Here's the drawing with two shaded views (mm, measured from the low corner). I have some questions. A direction names the side the tool comes from. Round coordinates to 2 decimals unless told otherwise and drop trailing zeros. Loops run counter-clockwise (first coordinate to the right, second up) from the corner with the lowest first, then second, coordinate; pieces in that order, holes last. Notation, with made-up numbers: (68, 36.25) -> (102, 36.25) arc R21 cw to (102, 41.25) -> close; hole circle Ø11 at (-17, 68.5). An arc over 180 degrees is marked (long way). Use a Markdown table: item, result.
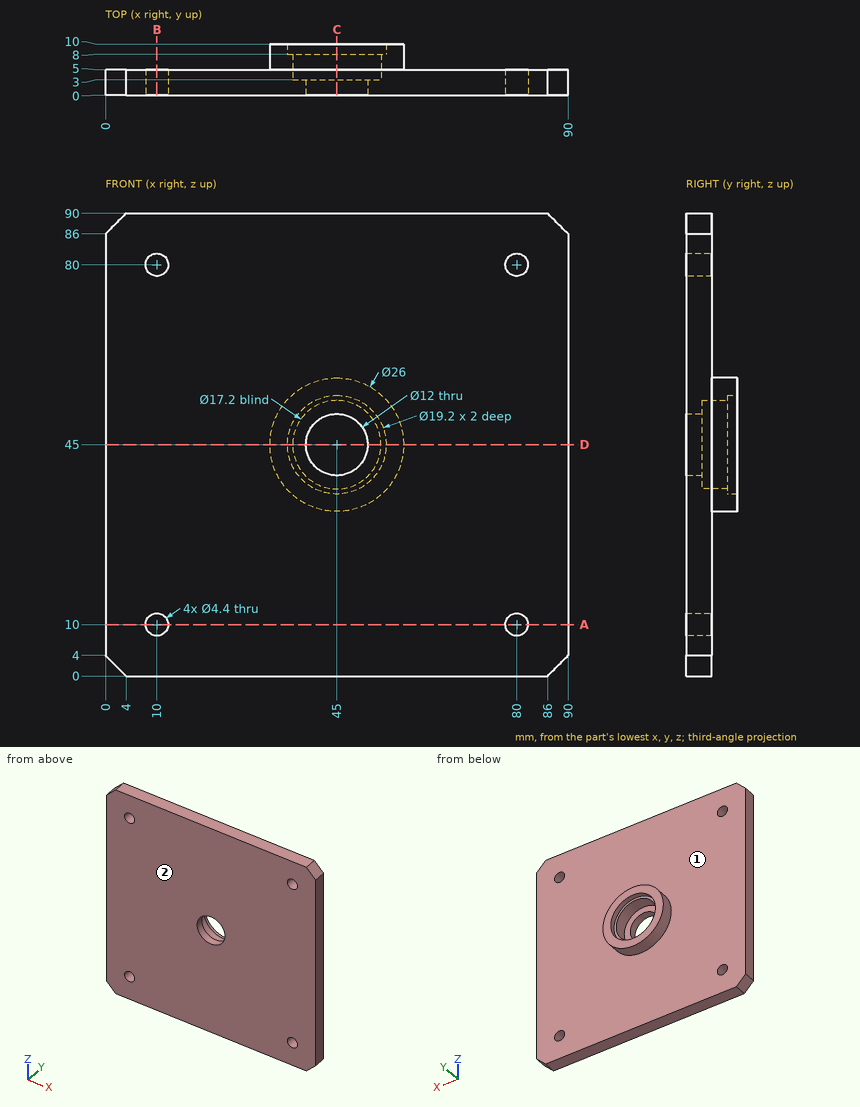
1. I want a section at A-A (z = 10). Please give me the cut outline in (x, y).
Answer sheet:
| item | result |
|---|---|
| outline | (0, 0) -> (7.8, 0) -> (7.8, 5) -> (0, 5) -> close; (12.2, 0) -> (77.8, 0) -> (77.8, 5) -> (12.2, 5) -> close; (82.2, 0) -> (90, 0) -> (90, 5) -> (82.2, 5) -> close |
2. I want a section at C-C (x = 45). Please give me the cut outline in (y, z), plus the area to 3 significant figures.
Answer sheet:
| item | result |
|---|---|
| outline | (0, 0) -> (5, 0) -> (5, 32) -> (10, 32) -> (10, 35.4) -> (8, 35.4) -> (8, 36.4) -> (3, 36.4) -> (3, 39) -> (0, 39) -> close; (0, 51) -> (3, 51) -> (3, 53.6) -> (8, 53.6) -> (8, 54.6) -> (10, 54.6) -> (10, 58) -> (5, 58) -> (5, 90) -> (0, 90) -> close |
| area | 420 mm² |
3. Which directions (+Z, -Z, +X, -X, +Y, -Y) give clear straight access to the entire face, cutting with the end or side of a thin tool? Please do the marked faces 1 and 2.
Answer sheet:
| item | result |
|---|---|
| face 1 | +Y |
| face 2 | +Z, -Z, +X, -X, -Y |
4. I want a section at D-D (z = 45). Please give me the cut outline in (x, y), plus the area to 3 significant figures.
Answer sheet:
| item | result |
|---|---|
| outline | (0, 0) -> (39, 0) -> (39, 3) -> (36.4, 3) -> (36.4, 8) -> (35.4, 8) -> (35.4, 10) -> (32, 10) -> (32, 5) -> (0, 5) -> close; (51, 0) -> (90, 0) -> (90, 5) -> (58, 5) -> (58, 10) -> (54.6, 10) -> (54.6, 8) -> (53.6, 8) -> (53.6, 3) -> (51, 3) -> close |
| area | 420 mm² |
5. Will these pins go through, and if not, where does the flat tip stop? pin 1 Ø9.5 at (x, z) = (41, 46.5) entering from +Y; pin 2 Ø2 at (y, z) = (7.5, 69.5) entering from +X.
Answer sheet:
| item | result |
|---|---|
| pin 1 | stops at y = 8 |
| pin 2 | passes through |
6. I need wall thicknesses on line 1 (X direction, y = 2.7, z = 10); line 2 (X direction, y = 9.1, z = 45); line 3 (X direction, y = 2.2, z = 45). Which ranges of each line are inside material? Lowest first, please.
Answer sheet:
| item | result |
|---|---|
| line 1 | x = 0 to 7.8, 12.2 to 77.8, 82.2 to 90 |
| line 2 | x = 32 to 35.4, 54.6 to 58 |
| line 3 | x = 0 to 39, 51 to 90 |
7. I want a section at B-B (x = 10). Please give me the cut outline in (y, z).
Answer sheet:
| item | result |
|---|---|
| outline | (0, 0) -> (5, 0) -> (5, 7.8) -> (0, 7.8) -> close; (0, 12.2) -> (5, 12.2) -> (5, 77.8) -> (0, 77.8) -> close; (0, 82.2) -> (5, 82.2) -> (5, 90) -> (0, 90) -> close |
